Verification items for the finished model (mm, model axes). A direction names the side the tool comes from. Round coordinates to 2 decimals unless told otherwise and drop trailing zeros. Order: outer loops, then holes, each group sorted by start corner. A loop starts at its lowest first (then second) coordinate and runs counter-clockwise, first axis right, second up. Notation, with made-up numbers: M 47.5,67 L 104.5,67 A12 cw 104.5,83 Z; hole C -11.5,-4 d5. An arc over 180 degrees is marked long. Answer as a JSON object with one key per item and string values. Group by question number.
```python
from build123d import *

# Parameters (mm, degrees)
EXTRUDE_1_DEPTH     = 5
SKETCH_3_R          = 1.5
SKETCH_3_R_2        = 1.375
SKETCH_3_R_3        = 1
CUT_EXTRUDE_1_DEPTH = 114.61053585


with BuildPart() as part:
    # 草图1 → 凸台-拉伸1 (new body)
    with BuildSketch(Plane(origin=(0, 0, 0), x_dir=(1, 0, 0), z_dir=(0, 1, 0))):
        with BuildLine():
            Line((-25.929831279, 46.15942029), (34.070168721, 46.15942029))
            ThreePointArc((34.070168721, 46.15942029), (37.605702627, 44.694954196), (39.070168721, 41.15942029))
            Line((39.070168721, 41.15942029), (39.070168721, -8.84057971))
            Line((39.070168721, -8.84057971), (43.820168721, -8.84057971))
            ThreePointArc((43.820168721, -8.84057971), (45.234382283, -9.426366148), (45.820168721, -10.84057971))
            Line((45.820168721, -10.84057971), (45.820168721, -46.84057971))
            ThreePointArc((45.820168721, -46.84057971), (45.234382283, -48.254793273), (43.820168721, -48.84057971))
            Line((43.820168721, -48.84057971), (39.070168721, -48.84057971))
            Line((39.070168721, -48.84057971), (39.070168721, -98.84057971))
            ThreePointArc((39.070168721, -98.84057971), (37.605702627, -102.376113616), (34.070168721, -103.84057971))
            Line((34.070168721, -103.84057971), (-25.929831279, -103.84057971))
            ThreePointArc((-25.929831279, -103.84057971), (-29.465365185, -102.376113616), (-30.929831279, -98.84057971))
            Line((-30.929831279, -98.84057971), (-30.929831279, -48.84057971))
            Line((-30.929831279, -48.84057971), (-35.679831279, -48.84057971))
            ThreePointArc((-35.679831279, -48.84057971), (-37.094044841, -48.254793273), (-37.679831279, -46.84057971))
            Line((-37.679831279, -46.84057971), (-37.679831279, -10.84057971))
            ThreePointArc((-37.679831279, -10.84057971), (-37.094044841, -9.426366148), (-35.679831279, -8.84057971))
            Line((-35.679831279, -8.84057971), (-30.929831279, -8.84057971))
            Line((-30.929831279, -8.84057971), (-30.929831279, 41.15942029))
            ThreePointArc((-30.929831279, 41.15942029), (-29.465365185, 44.694954196), (-25.929831279, 46.15942029))
        make_face()
    extrude(amount=EXTRUDE_1_DEPTH)

    # 草图3 → 切除-拉伸1 (cut, through all)
    with BuildSketch(Plane(origin=(0, 5, 0), x_dir=(1, 0, 0), z_dir=(0, 1, 0))):
        with Locations(Location((34.070168721, 41.15942029, 0), (0, 0, 270))):
            Circle(SKETCH_3_R)
        with Locations(Location((-25.929831279, 41.15942029, 0), (0, 0, 270))):
            Circle(SKETCH_3_R)
        with Locations(Location((-25.929831279, -98.84057971, 0), (0, 0, 270))):
            Circle(SKETCH_3_R)
        with Locations(Location((34.070168721, -98.84057971, 0), (0, 0, 270))):
            Circle(SKETCH_3_R)
        with Locations(Location((34.070168721, -28.84057971, 0), (0, 0, 270))):
            Circle(SKETCH_3_R)
        with Locations(Location((-25.929831279, -28.84057971, 0), (0, 0, 270))):
            Circle(SKETCH_3_R)
        with Locations(Location((26.570168721, -31.962567588, 0), (0, 0, 270))):
            Circle(SKETCH_3_R_2)
        with Locations(Location((-22.429831279, -31.962567588, 0), (0, 0, 270))):
            Circle(SKETCH_3_R_2)
        with Locations(Location((26.570168721, -89.962567588, 0), (0, 0, 270))):
            Circle(SKETCH_3_R_2)
        with Locations(Location((-22.429831279, -89.962567588, 0), (0, 0, 270))):
            Circle(SKETCH_3_R_2)
        with Locations(Location((-10.179831279, 40.658771251, 0), (0, 0, 270))):
            Circle(SKETCH_3_R_3)
        with Locations(Location((18.320168721, 40.658771251, 0), (0, 0, 90))):
            Circle(SKETCH_3_R_3)
        with Locations(Location((-10.179831279, 8.158771251, 0), (0, 0, 90))):
            Circle(SKETCH_3_R_3)
        with Locations(Location((18.320168721, 8.158771251, 0), (0, 0, 270))):
            Circle(SKETCH_3_R_3)
    extrude(amount=-CUT_EXTRUDE_1_DEPTH, mode=Mode.SUBTRACT)


solid = part.part
```
Q1. Cross-section at A-A, the plane y = 1.7. Give the number of separate pieces and of enclosed holes in the cut face, then the cut area to 3 significant figures.
Q2. Thickness scan on line 1 (X direction, y = 1.85, z = 29); line 2 (X direction, y = 0.75, z = 8); line 3 (Z direction, x = -21.5, y = 3.4). Record the ranges inside material, lowest first. Write a range as from..to.
Q3. Gauge pin test, flat ends, axial feed: pin 1 Ø2.5 at (x, y) = (40.5, 3) entering from +Z; pin 2 Ø1.8 at (x, z) = (-25.93, 28.84) entering from -Y; pin 3 Ø1.5 at (y, z) = (2, -25.5) entering from -X. Record the tip position at first contact, or that the pin passes through.
Q4. Cross-section at B-B, the plane z = -23. Record the cut outline in (x, y), then the cut area to 3 significant figures.
Q5. Tool access check on faces 5 (the face through (41, 2, 8.841)), 6 (the face through (39.07, 2, 73)), 7 (the face through (-30.93, 2, -16)), 8 (the face through (-30.93, 2, 74)), 9 (the face through (27.73, 2.54, 90.7)). Record the directions out of +Z, -Z, +X, -X, +Y, -Y that give a thin tool (end or side, any length) a straight path to the whole face; none if there is none.
Q6. Release check for a two-part mould opening along Z. For faces 1 (the face through (-21.27, 2.54, 90.7)), 2 (the face through (27.73, 2.54, 32.7)), 3 (the face through (37.64, 2.46, 102.34)), 4 (the face through (-33, 2, 8.841)) record: released by +Z, released by -Z, zero draft, split by the parting line, or undercut.
Conclusion:
{
 "1": {"separate pieces": "1", "enclosed holes": "14", "area": "10,900 mm2"},
 "2": {"line 1": "-37.68..-27.42, -24.44..32.58, 35.56..45.82", "line 2": "-30.93..39.07", "line 3": "-46.16..30.95, 32.98..88.95, 90.98..103.84"},
 "3": {"pin 1": "z = 48.84", "pin 2": "through", "pin 3": "x = -30.93"},
 "4": {"outline": "M -30.93,0 L 39.07,0 L 39.07,5 L -30.93,5 Z", "area": "350 mm2"},
 "5": {"face 5": "-Z, +X, +Y, -Y", "face 6": "+Z, +X, +Y, -Y", "face 7": "-Z, -X, +Y, -Y", "face 8": "+Z, -X, +Y, -Y", "face 9": "+Y, -Y"},
 "6": {"face 1": "undercut", "face 2": "undercut", "face 3": "released by +Z", "face 4": "released by -Z"}
}
